The model under review builds one solid part; all positions refer to its coordinate system, in mm. Face numbers are marked on the shaded views. Give positions to 0.01 mm unless a question says otherwise; leave off trailing zeros. Order: outer loops, then holes, each group sorted by start corner. A loop starts at its lowest first (then second) coordinate and runs counter-clockwise, first axis right, second up. Notation, with made-up numbers: (36, 87) - (47, 87) arc R17 cw to (47, 108) - close; hole circle Ø8 at (24, -27.75). An arc over 180 degrees is marked (long way). Use CSV: the item, a comma, the result in double quotes. Start each with the question number.
1. To check wall thickness, follow line 1 (Z direction, x = -34.65, y = 4.45); line 2 (X direction, y = 1.7, z = -92.45); line 3 (X direction, y = 8.75, z = -27). State the ranges of each line that lie inside material, in increasing order. Write a range as [from, to].
2. Draft analysis for pull direction Y (two halves, no side actions). For the marked faces 1 and 2, state which applies: released by +Y, released by -Y, zero draft, split by the parting line, or undercut.
3. For pin 1 (1.2 mm diameter, centred on y = 4, z = -206, fed in from +X); pin 2 (3 mm diameter, centred on x = 1.5, y = 9, fed in from +Z); pin 3 (3 mm diameter, centred on x = -34.65, z = -92.45, fed in from -Y), all flat-tipped, find the tip position at first contact; note any pin that passes through.
4. Take a section at B-B, the plane z = -51. State the section outline as (x, y) points.
5. Take a section at A-A, the plane x = -85. State the section outline as (y, z) points.
Autodesk Inventor part; units mm, degrees
ref_plane "YZ Plane" through (0, 0, 0) normal (1, 0, 0) x (0, 1, 0)
ref_plane "XZ Plane" through (0, 0, 0) normal (0, 1, 0) x (-1, 0, 0)
ref_plane "XY Plane" through (0, 0, 0) normal (0, 0, 1) x (1, 0, 0)
sketch "Sketch1" plane through (0, 0, 0) normal (0, 1, 0) x (-1, 0, 0)
  line L0 (0, 0) -> (-120, 0)
  line L1 (-120, 0) -> (-120, -226)
  line L2 (-120, -226) -> (0, -226)
  line L3 (0, -226) -> (0, 0)
  dimension "d0" = 120
  dimension "d1" = 226
extrude "Extrusion1" add sketch "Sketch1" along normal blind 10
sketch "Sketch2" plane through (120, 0, 0) normal (1, 0, 0) x (0, 0, -1)
  circle A0 centre (30, 5) radius 2
  line L0 (0, 0) -> (0, 10)
  line L1 (0, 10) -> (226, 10)
  circle A1 centre (206, 5) radius 2
  dimension "d4" = 4
  dimension "d5" = 30
  dimension "d6" = 5
  dimension "d9" = 176
extrude "Extrusion2" cut sketch "Sketch2" against normal blind 10
sketch "Sketch3" plane through (0, 0, 0) normal (0, 0, 1) x (1, 0, 0)
  circle A0 centre (20, 5) radius 2
  line L0 (0, 10) -> (120, 10)
  line L1 (0, 0) -> (0, 10)
  dimension "d16" = 4
  dimension "d17" = 5
  dimension "d18" = 20
extrude "Extrusion3" cut sketch "Sketch3" against normal blind 10
mirror "Mirror1" about plane through (0, 0, -226) normal (-1, 0, 0)
sketch "Sketch4" plane through (0, 10, 0) normal (0, 1, 0) x (1, 0, 0)
  circle A0 centre (0, 97.45) radius 10
  line L0 (120, 0) -> (-120, 0)
  line L1 (-30.1, 107.45) -> (10.4, 107.45)
  line L2 (10.4, 107.45) -> (10.4, 87.45)
  line L3 (10.4, 87.45) -> (-30.1, 87.45)
  line L4 (-30.1, 87.45) -> (-30.1, 107.45)
  circle A1 centre (-34.65, 92.45) radius 1.75
  circle A2 centre (-34.65, 102.45) radius 1.75
  circle A3 centre (15.85, 92.45) radius 1.75
  circle A4 centre (15.85, 102.45) radius 1.75
  arc A5 (10.4, 107.45) -> (8.4, 107.45) centre (9.4, 107.45) ccw
  arc A6 (8.4, 87.45) -> (10.4, 87.45) centre (9.4, 87.45) ccw
  arc A7 (-28.1, 107.45) -> (-30.1, 107.45) centre (-29.1, 107.45) ccw
  arc A8 (-30.1, 87.45) -> (-28.1, 87.45) centre (-29.1, 87.45) ccw
  arc A9 (-90, 30) -> (-80, 30) centre (-85, 30) ccw
  arc A10 (-80, 60) -> (-90, 60) centre (-85, 60) ccw
  line L5 (-90, 30) -> (-90, 60)
  line L6 (-80, 30) -> (-80, 60)
  line L7 (-120, 0) -> (-120, 226)
  point P0 (0, 0)
  dimension "d21" = 97.45
  dimension "d22" = 0
  dimension "d23" = 20
  dimension "d24" = 20
  dimension "d27" = 10.4
  dimension "d28" = 3.5
  dimension "d31" = 10
  dimension "d34" = 50.5
  dimension "d37" = 5
  dimension "d38" = 4.55
  dimension "d39" = 30.1
  dimension "d50" = 1
  dimension "d54" = 10
  dimension "d55" = 30
  dimension "d56" = 30
  dimension "d57" = 30
extrude "Extrusion4" cut sketch "Sketch4" against normal through all
sketch "Sketch5" plane through (0, 10, 0) normal (0, 1, 0) x (1, 0, 0)
  line L0 (-37.1, 112.45) -> (17.4, 112.45)
  line L1 (20.4, 109.45) -> (20.4, 85.45)
  line L2 (17.4, 82.45) -> (-37.1, 82.45)
  line L3 (-40.1, 85.45) -> (-40.1, 109.45)
  line L4 (10.4, 107.45) -> (10.4, 87.45)
  line L5 (-28.1, 107.45) -> (8.4, 107.45)
  arc A0 (-40.1, 85.45) -> (-37.1, 82.45) centre (-37.1, 85.45) ccw
  arc A1 (-37.1, 112.45) -> (-40.1, 109.45) centre (-37.1, 109.45) ccw
  arc A2 (20.4, 109.45) -> (17.4, 112.45) centre (17.4, 109.45) ccw
  arc A3 (17.4, 82.45) -> (20.4, 85.45) centre (17.4, 85.45) ccw
  point P0 (0, 0)
  point P1 (-40.1, 112.45)
  point P2 (20.4, 82.45)
  point P3 (20.4, 112.45)
  point P4 (-40.1, 82.45)
  point P5 (-30.1, 107.45)
  dimension "d42" = 10
  dimension "d43" = 30
  dimension "d44" = 60.5
  dimension "d45" = 5
  dimension "d48" = 3
extrude "Extrusion5" cut sketch "Sketch5" against normal blind 4
sketch "Sketch6" plane through (0, 10, 0) normal (0, 1, 0) x (1, 0, 0)
  line L0 (-10, 0) -> (10, 0)
  line L1 (10, 0) -> (10, 57)
  line L2 (7, 60) -> (-7, 60)
  line L3 (-10, 57) -> (-10, 0)
  line L4 (120, 0) -> (-120, 0)
  arc A0 (-7, 60) -> (-10, 57) centre (-7, 57) ccw
  arc A1 (10, 57) -> (7, 60) centre (7, 57) ccw
  point P0 (0, 0)
  point P1 (10, 60)
  point P2 (-10, 60)
  dimension "d58" = 20
  dimension "d59" = 60
  dimension "d60" = 10
  dimension "d61" = 0
  dimension "d64" = 3
extrude "Extrusion6" cut sketch "Sketch6" against normal blind 6
sketch "Sketch7" plane through (0, 4, 0) normal (0, 1, 0) x (1, 0, 0)
  line L0 (-10, 0) -> (-10, 57)
  line L1 (-10, 0) -> (10, 0)
  line L2 (10, 0) -> (10, 3)
  line L3 (7, 6) -> (-7, 6)
  line L4 (-10, 3) -> (-10, 0)
  arc A0 (-7, 6) -> (-10, 3) centre (-7, 3) ccw
  arc A1 (10, 3) -> (7, 6) centre (7, 3) ccw
  point P0 (0, 0)
  point P1 (10, 6)
  point P2 (-10, 6)
  dimension "d66" = 20
  dimension "d67" = 6
  dimension "d70" = 3
extrude "Extrusion7" cut sketch "Sketch7" against normal through all
equation "\"d4\" = screws"
equation "\"d16\" = screws"
equation "\"screws\" = 4"
properties part number "box_shelf"
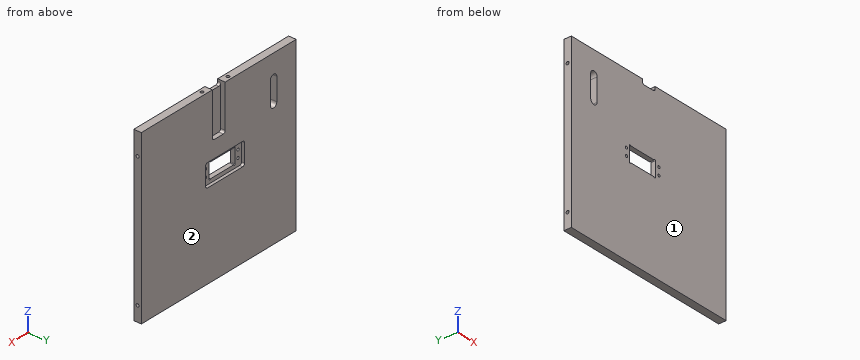
Determined:
1,line 1,"z = [-226, -104.2], [-100.7, -94.2], [-90.7, 0]"
1,line 2,"x = [-120, -36.4], [-32.9, -30.1], [10.4, 14.1], [17.6, 120]"
1,line 3,"x = [-120, -89], [-81, -10], [10, 120]"
2,face 1,"released by -Y"
2,face 2,"released by +Y"
3,pin 1,"stops at x = 110"
3,pin 2,"stops at z = -60"
3,pin 3,"passes through"
4,outline,"(-120, 0) - (-90, 0) - (-90, 10) - (-120, 10) - close; (-80, 0) - (120, 0) - (120, 10) - (10, 10) - (10, 4) - (-10, 4) - (-10, 10) - (-80, 10) - close"
5,outline,"(0, -226) - (10, -226) - (10, -65) - (0, -65) - close; (0, -25) - (10, -25) - (10, 0) - (0, 0) - close"
